Verification items for the finished model (mm, model axes). Face numbers are marked on the shaded views. Coordinates: 2 decimals unless noted, no trailing zeros. Write each loop counter-clockwise with the first axis right and the second up, starting at its lowest first coordinate (ties: lowest second). Pieces come first, ordered by that corner, then holes. Notation, with made-up numbers: (76.25, -2.5) - (122.25, -2.5) arc R25 cw to (122.25, 25.5) - close; hole circle Ø7 at (-11.75, 5.5). An arc over 180 degrees is marked (long way). Use CSV: the item, a comma, the result in double quotes. Start each with the question number.
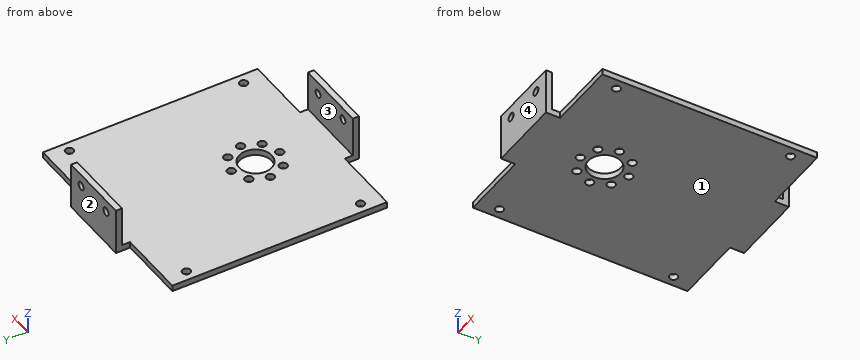
```python
from build123d import *

# Parameters (mm, degrees)
F0_W     = 18
F0_H     = 60
F0_R     = 1
F0_R_2   = 4
F1_DEPTH = 1.5
F2_W     = 18
F2_H     = 1.5
F3_DEPTH = 10
F4_R     = 1
F5_DEPTH = 60.001
F6_W     = 53
F6_H     = 1.5
F7_DEPTH = 17
F8_R     = 1
F9_DEPTH = 1.5


with BuildPart() as f1:
    # F0 (on Top) → F1 (new body)
    with BuildSketch(Plane.XY):
        with Locations((0, 10)):
            Rectangle(F0_W, F0_H)
        with Locations((-6, 0)):
            Circle(F0_R, mode=Mode.SUBTRACT)
        with Locations((-4.242641, -4.242641)):
            Circle(F0_R, mode=Mode.SUBTRACT)
        with Locations((-4.242641, 4.242641)):
            Circle(F0_R, mode=Mode.SUBTRACT)
        with Locations((0, -6)):
            Circle(F0_R, mode=Mode.SUBTRACT)
        Circle(F0_R_2, mode=Mode.SUBTRACT)
        with Locations((4.242641, -4.242641)):
            Circle(F0_R, mode=Mode.SUBTRACT)
        with Locations((0, 6)):
            Circle(F0_R, mode=Mode.SUBTRACT)
        with Locations((4.242641, 4.242641)):
            Circle(F0_R, mode=Mode.SUBTRACT)
        with Locations((6, 0)):
            Circle(F0_R, mode=Mode.SUBTRACT)
    extrude(amount=F1_DEPTH)

    # F2 (on face) → F3 (join)
    with BuildSketch(Plane.XY.offset(1.5)):
        with Locations((0, 39.25)):
            Rectangle(F2_W, F2_H)
        with Locations((0, -19.25)):
            Rectangle(F2_W, F2_H)
    extrude(amount=F3_DEPTH)

    # F4 (on face) → F5 (cut, through all)
    with BuildSketch(Plane.XZ.offset(20)):
        with Locations((5, 8.5)):
            Circle(F4_R)
        with Locations((-5, 8.5)):
            Circle(F4_R)
    extrude(amount=-F5_DEPTH, mode=Mode.SUBTRACT)

    # F6 (on face) → F7 (join)
    with BuildSketch(Plane.YZ.offset(9)):
        with Locations((10, 0.75)):
            Rectangle(F6_W, F6_H)
    extrude(amount=F7_DEPTH)

    # F8 (on face) → F9 (cut, through all)
    with BuildSketch(Plane.XY.offset(1.5)):
        with Locations((23.5, 31.5)):
            Circle(F8_R)
        with Locations((23.5, -11.5)):
            Circle(F8_R)
    extrude(amount=-F9_DEPTH, mode=Mode.SUBTRACT)

    # F10: F1 across plane


with BuildPart() as f1_1:
    add(f1.part)
    add(f1.part.mirror(Plane.YZ))


solid = f1_1.part
```
Q1. Release check for a two-part mould opening along Y. For the marked faces 1, 2, 3 and 4 record: released by +Y, released by -Y, zero draft, split by the parting line, or undercut.
Q2. Cross-section at D-D (y = 31.5). Record the cut outline in (x, z).
Q3. Scan lines: line 1 along Y through (x, z) = (23.5, 0.65); line 2 along X through (y, z) = (39.3, 8.5); line 3 along X through (y, z) = (0, 0.9). Record each from-to range of solid material in increasing order. Write a range as from..to.
Q4. Gauge pin test, flat ends, axial feed: pin 1 (2 mm diameter, centred on x = -14, y = 20, fed in from +Z); pin 2 (4 mm diameter, centred on y = -18.5, z = 5, fed in from +X); pin 3 (1.6 mm diameter, centred on x = -19, z = 0.5, fed in from +Y). Record the tip position at first contact, or that the pin passes through.
Q5. Cross-section at B-B (y = 0). Record the cut outline in (x, z), plus the area to 3 significant figures.
Q6. Cross-section at A-A (y = -6). Record the cut outline in (x, z), plus the area to 3 significant figures.
Q7. Cross-section at C-C (z = 5). Record the cut outline in (x, y).
Reply:
1,face 1,"zero draft"
1,face 2,"released by +Y"
1,face 3,"undercut"
1,face 4,"released by -Y"
2,outline,"(-26, 0) - (-24.5, 0) - (-24.5, 1.5) - (-26, 1.5) - close; (-22.5, 0) - (22.5, 0) - (22.5, 1.5) - (-22.5, 1.5) - close; (24.5, 0) - (26, 0) - (26, 1.5) - (24.5, 1.5) - close"
3,line 1,"-16.5..-12.5, -10.5..30.5, 32.5..36.5"
3,line 2,"-9..-6, -4..4, 6..9"
3,line 3,"-26..-7, -5..-4, 4..5, 7..26"
4,pin 1,"z = 1.5"
4,pin 2,"x = 9"
4,pin 3,"y = 36.5"
5,outline,"(-26, 0) - (-7, 0) - (-7, 1.5) - (-26, 1.5) - close; (-5, 0) - (-4, 0) - (-4, 1.5) - (-5, 1.5) - close; (4, 0) - (5, 0) - (5, 1.5) - (4, 1.5) - close; (7, 0) - (26, 0) - (26, 1.5) - (7, 1.5) - close"
5,area,"60.0 mm^2"
6,outline,"(-26, 0) - (-1, 0) - (-1, 1.5) - (-26, 1.5) - close; (1, 0) - (26, 0) - (26, 1.5) - (1, 1.5) - close"
6,area,"75.0 mm^2"
7,outline,"(-9, -20) - (9, -20) - (9, -18.5) - (-9, -18.5) - close; (-9, 38.5) - (9, 38.5) - (9, 40) - (-9, 40) - close"
